The model under review builds one solid part; all positions refer to its coordinate system, in mm. A direction names the side the tool comes from. Coordinates: 2 decimals unless noted, no trailing zeros. Write each loop counter-clockwise with the first axis right and the second up, starting at its lowest first coordinate (ties: lowest second). Pieces come first, ordered by that corner, then holes. Notation, with made-up numbers: (4.5, 78) - (44.5, 78) arc R18 cw to (44.5, 95) - close; hole circle Ø7 at (21.25, 16). An arc over 180 degrees is marked (long way). Put each result on its own line as item: value.
from build123d import *

# Parameters (mm, degrees)
SKETCH2_W            = 18
SKETCH2_H            = 18
BOSS_EXTRUDE1_DEPTH  = 2
SKETCH3_W            = 18
SKETCH3_H            = 2
BOSS_EXTRUDE2_DEPTH  = 8
SKETCH4_W            = 18
SKETCH4_H            = 2
BOSS_EXTRUDE3_DEPTH  = 12
BOSS_EXTRUDE4_DEPTH  = 8
SKETCH6_W            = 9.8
SKETCH6_H            = 2
BOSS_EXTRUDE5_DEPTH  = 5
SKETCH6_2_W          = 9.8
SKETCH6_2_H          = 2
BOSS_EXTRUDE7_DEPTH  = 5
SKETCH9_W            = 5
SKETCH9_H            = 9.8
BOSS_EXTRUDE8_DEPTH  = 9.8
SKETCH10_W           = 10
SKETCH10_H           = 8
CUT_EXTRUDE2_DEPTH   = 11.8
SKETCH11_W           = 2
SKETCH11_H           = 8
CUT_EXTRUDE4_DEPTH   = 8
SKETCH16_W           = 8
SKETCH16_H           = 8
CUT_EXTRUDE5_DEPTH   = 8
SKETCH17_W           = 2
SKETCH17_H           = 8
BOSS_EXTRUDE11_DEPTH = 8
SKETCH18_W           = 2
SKETCH18_H           = 8
CUT_EXTRUDE6_DEPTH   = 8


with BuildPart() as part:
    # Sketch2 → Boss-Extrude1 (new body)
    with BuildSketch(Plane(origin=(0, 0, 0), x_dir=(1, 0, 0), z_dir=(0, 1, 0))):
        Rectangle(SKETCH2_W, SKETCH2_H)
    extrude(amount=BOSS_EXTRUDE1_DEPTH)

    # Sketch3 → Boss-Extrude2 (add)
    with BuildSketch(Plane.XZ):
        with Locations((0, 8)):
            Rectangle(SKETCH3_W, SKETCH3_H)
        with Locations((0, -8)):
            Rectangle(SKETCH3_W, SKETCH3_H)
    extrude(amount=BOSS_EXTRUDE2_DEPTH)

    # Sketch4 → Boss-Extrude3 (add)
    with BuildSketch(Plane(origin=(9, 0, 0), x_dir=(0, 0, -1), z_dir=(1, 0, 0))):
        with Locations((0, 1)):
            Rectangle(SKETCH4_W, SKETCH4_H)
    extrude(amount=BOSS_EXTRUDE3_DEPTH)

    # Sketch5 → Boss-Extrude4 (add)
    with BuildSketch(Plane.XZ):
        Polygon((21, 9), (19, 9), (9, 9), (9, 7), (19, 7), (19, -9), (21, -9), align=None)
    extrude(amount=BOSS_EXTRUDE4_DEPTH)

    # Sketch6 → Boss-Extrude5 (add)
    with BuildSketch(Plane.ZY.offset(9)):
        with Locations((0, 1)):
            Rectangle(SKETCH6_W, SKETCH6_H)
    extrude(amount=BOSS_EXTRUDE5_DEPTH)

    # Sketch6<2> → Boss-Extrude7 (add)
    with BuildSketch(Plane.ZY.offset(9)):
        with Locations((0, 1)):
            Rectangle(SKETCH6_2_W, SKETCH6_2_H)
    extrude(amount=BOSS_EXTRUDE7_DEPTH)

    # Sketch9 → Boss-Extrude8 (add)
    with BuildSketch(Plane(origin=(0, 2, 0), x_dir=(1, 0, 0), z_dir=(0, 1, 0))):
        with Locations((-11.5, 0)):
            Rectangle(SKETCH9_W, SKETCH9_H)
    extrude(amount=BOSS_EXTRUDE8_DEPTH)

    # Sketch10 → Cut-Extrude2 (cut)
    with BuildSketch(Plane(origin=(0, 0, 7), x_dir=(-1, 0, 0), z_dir=(0, 0, -1))):
        with Locations((-14, -4)):
            Rectangle(SKETCH10_W, SKETCH10_H)
    extrude(amount=-CUT_EXTRUDE2_DEPTH, mode=Mode.SUBTRACT)

    # Sketch11 → Cut-Extrude4 (cut)
    with BuildSketch(Plane.ZY.offset(9)):
        with Locations((-8, -4)):
            Rectangle(SKETCH11_W, SKETCH11_H)
    extrude(amount=-CUT_EXTRUDE4_DEPTH, mode=Mode.SUBTRACT)

    # Sketch16 → Cut-Extrude5 (cut)
    with BuildSketch(Plane(origin=(0, 0, 7), x_dir=(-1, 0, 0), z_dir=(0, 0, -1))):
        with Locations((5, -4)):
            Rectangle(SKETCH16_W, SKETCH16_H)
    extrude(amount=-CUT_EXTRUDE5_DEPTH, mode=Mode.SUBTRACT)

    # Sketch17 → Boss-Extrude11 (add)
    with BuildSketch(Plane.ZY.offset(1)):
        with Locations((-8, -4)):
            Rectangle(SKETCH17_W, SKETCH17_H)
        with Locations((8, -4)):
            Rectangle(SKETCH17_W, SKETCH17_H)
    extrude(amount=BOSS_EXTRUDE11_DEPTH)

    # Sketch18 → Cut-Extrude6 (cut)
    with BuildSketch(Plane(origin=(9, 0, 0), x_dir=(0, 0, -1), z_dir=(1, 0, 0))):
        with Locations((8, -4)):
            Rectangle(SKETCH18_W, SKETCH18_H)
        with Locations((-8, -4)):
            Rectangle(SKETCH18_W, SKETCH18_H)
    extrude(amount=-CUT_EXTRUDE6_DEPTH, mode=Mode.SUBTRACT)


solid = part.part
1. Consider section B-B on x = -7. State the section outline as (y, z) points.
Determined:
outline: (-8, -9) - (2, -9) - (2, 9) - (-8, 9) - (-8, 7) - (0, 7) - (0, -7) - (-8, -7) - close
2. To check wall thickness, follow probe 1 along X at (y, z) = (-1.75, -8); probe 2 along Y at (x, z) = (6, 1); probe 3 along X at (y, z) = (-1.75, 5). State the ranges of each line that lie inside material, in increasing order.
Determined:
probe 1: x = -9 to 1, 19 to 21
probe 2: y = 0 to 2
probe 3: x = 19 to 21
3. Consider section A-A on z = 3. State the section outline as (x, y) points.
Determined:
outline: (-14, 0) - (19, 0) - (19, -8) - (21, -8) - (21, 2) - (-9, 2) - (-9, 11.8) - (-14, 11.8) - close
4. Consider section C-C on y = 9.25. State the section outline as (x, z) points.
Determined:
outline: (-14, -4.9) - (-9, -4.9) - (-9, 4.9) - (-14, 4.9) - close
5. For pin 1 Ø1.5 at (x, z) = (-1, -1) entering from +Y; pin 2 Ø5.5 at (x, y) = (-10.5, 7) entering from +Z; pin 3 Ø6 at (x, y) = (5.5, 7) entering from +Z; pin 4 Ø6.5 at (y, z) = (-3.5, 0) entering from -X, all flat-tipped, find the tip position at first contact; note any pin that passes through.
Determined:
pin 1: stops at y = 2
pin 2: stops at z = 4.9
pin 3: passes through
pin 4: stops at x = 19
6. Machinability: for faces 1 (the flat face through (-4, -4, -7)), 2 (the flat face through (19, -4, 0)), 3 (the flat face through (-9, -2, -8)), 4 (the flat face through (-9, 7, 0)), which of the approach directions +Z, -Z, +X, -X, +Y, -Y give a long, thin tool a straight path to every point of the face, cutting with its end or side? Answer none if there is none.
Determined:
face 1: -X, -Y
face 2: +Z, -Z, -Y
face 3: -Z, -X, +Y, -Y
face 4: +Z, -Z, +X, +Y
7. The part is to be moulded in two halves that separate along Z. For faces 5 (the flat face through (-4, -4, 7)), 6 (the flat face through (-12, 6, -4.9)), 7 (the flat face through (2.9, 0.4, 9)), say which applies: +Z half, -Z half, draft (parallel to the pull), parting line (faces both ways), or undercut.
Determined:
face 5: undercut
face 6: -Z half
face 7: +Z half
8. Consider section D-D on z = -6. State the section outline as (x, y) points, plus the area to 3 significant figures.
Determined:
outline: (-9, 0) - (19, 0) - (19, -8) - (21, -8) - (21, 2) - (-9, 2) - close
area: 76.0 mm^2
